```python
from build123d import *

# Parameters (mm, degrees)
F1_DEPTH = 12.7
F2_R     = 5.08


with BuildPart() as f1:
    # F0 (on Front) → F1 (new body, symmetric)
    with BuildSketch(Plane.XZ):
        with BuildLine():
            Line((58.801, 25.4), (58.801, 3.175))
            ThreePointArc((58.801, 3.175), (61.046064, 2.245064), (61.976, 0))
            ThreePointArc((61.976, 0), (61.046064, -2.245064), (58.801, -3.175))
            Line((58.801, -3.175), (58.801, -25.4))
            ThreePointArc((58.801, -25.4), (84.201, 0), (58.801, 25.4))
        make_face()
        with BuildLine():
            Line((-55.626, 0), (0, 0))
            Line((0, 0), (55.626, 0))
            ThreePointArc((55.626, 0), (56.555936, 2.245064), (58.801, 3.175))
            Line((58.801, 3.175), (58.801, 25.4))
            Line((58.801, 25.4), (-58.801, 25.4))
            Line((-58.801, 25.4), (-58.801, 3.175))
            ThreePointArc((-58.801, 3.175), (-56.555936, 2.245064), (-55.626, 0))
        make_face()
        with BuildLine():
            Line((55.626, 0), (0, 0))
            Line((0, 0), (-55.626, 0))
            ThreePointArc((-55.626, 0), (-56.555936, -2.245064), (-58.801, -3.175))
            Line((-58.801, -3.175), (-58.801, -25.4))
            Line((-58.801, -25.4), (58.801, -25.4))
            Line((58.801, -25.4), (58.801, -3.175))
            ThreePointArc((58.801, -3.175), (56.555936, -2.245064), (55.626, 0))
        make_face()
        with BuildLine():
            ThreePointArc((-58.801, -3.175), (-61.976, 0), (-58.801, 3.175))
            Line((-58.801, 3.175), (-58.801, 25.4))
            ThreePointArc((-58.801, 25.4), (-84.201, 0), (-58.801, -25.4))
            Line((-58.801, -25.4), (-58.801, -3.175))
        make_face()
    extrude(amount=F1_DEPTH, both=True)

    # F2
    f2_edges = [f1.edges().sort_by_distance(p)[0] for p in [
        (-84.201, -12.7, 0),
        (0, -12.7, 25.4),
    ]]
    fillet(f2_edges, radius=F2_R)


solid = f1.part
```
The model under review builds one solid part; all positions refer to its coordinate system, in mm. Round coordinates to 2 decimals unless told otherwise and drop trailing zeros. Loops run counter-clockwise (first coordinate to the right, second up) from the corner with the lowest first, then second, coordinate; pieces in that order, holes last. Notation, with made-up numbers: (54, 35.25) -> (108, 35.25) arc R29 cw to (108, 64.25) -> close; hole circle Ø3 at (-17, -22.5). An arc over 180 degrees is marked (long way). Answer as a JSON object with one key per item and string values. Group by question number.
1) We need section A-A on y = 6.75. Write out the cut boundary in (x, z) (3 decimals), then the cut area to 3 significant figures.
2) For pin 1 Ø3 at (y, z) = (4.5, -7.5) entering from -X; pin 2 Ø1 at (y, z) = (-9, -4.5) entering from +X, all flat-tipped, find the tip position at first contact; note any pin that passes through.
3) We need section B-B on y = -9.75. Write out the cut boundary in (x, z) (3 decimals).
4) For line 1 (X direction, y = 10.5, z = -1.5); line 2 (X direction, y = 7, z = 2); line 3 (Z direction, x = -58, y = 4.5), list the stretches that pass through material, from the lowest coordinate up. Write a range as [from, to].
Result set:
{
 "1": {"outline": "(-58.801, -25.4) -> (58.801, -25.4) arc R25.4 ccw to (58.801, 25.4) -> (-58.801, 25.4) arc R25.4 ccw to start; hole circle Ø6.35 at (-58.801, 0); hole circle Ø6.35 at (58.801, 0)", "area": "7,940 mm²"},
 "2": {"pin 1": "x = -83.48", "pin 2": "x = 83.75"},
 "3": {"outline": "(-58.801, -24.932) -> (58.801, -24.932) arc R24.932 ccw to (58.801, 24.932) -> (-58.801, 24.932) arc R24.932 ccw to start; hole circle Ø6.35 at (-58.801, 0); hole circle Ø6.35 at (58.801, 0)"},
 "4": {"line 1": "[-84.16, -61.6], [-56, 56], [61.6, 84.16]", "line 2": "[-84.12, -61.27], [-56.34, 56.34], [61.27, 84.12]", "line 3": "[-25.4, -3.07], [3.07, 25.4]"}
}
